```python
from build123d import *

# Parameters (mm, degrees)
SKETCH1_W           = 27
SKETCH1_H           = 10
BOSS_EXTRUDE1_DEPTH = 10
FILLET1_R           = 4
SKETCH4_R           = 8.2
CUT_EXTRUDE3_DEPTH  = 18.528548143
BOSS_EXTRUDE2_START = 2
BOSS_EXTRUDE2_DEPTH = 5.4
SKETCH2_R           = 1.7
CUT_EXTRUDE1_DEPTH  = 20.551214796
SKETCH3_R           = 3
CUT_EXTRUDE2_DEPTH  = 3


with BuildPart() as part:
    # Sketch1 → Boss-Extrude1 (new body)
    with BuildSketch(Plane.XY):
        Rectangle(SKETCH1_W, SKETCH1_H)
    extrude(amount=BOSS_EXTRUDE1_DEPTH)

    # Fillet1
    fillet1_edges = [part.edges().sort_by_distance(p)[0] for p in [
        (-13.5, 0, 10),
        (13.5, 0, 10),
        (-13.5, 0, 0),
        (13.5, 0, 0),
    ]]
    fillet(fillet1_edges, radius=FILLET1_R)

    # Sketch4 → Cut-Extrude3 (cut, through all)
    with BuildSketch(Plane(origin=(0, 0, 0), x_dir=(-1, 0, 0), z_dir=(0, 0, -1))):
        with Locations((0, -5)):
            Circle(SKETCH4_R)
    extrude(amount=-CUT_EXTRUDE3_DEPTH, mode=Mode.SUBTRACT)

    # Sketch5 → Boss-Extrude2 (add)
    with BuildSketch(Plane.XY.offset(BOSS_EXTRUDE2_START)):
        with BuildLine():
            Line((8.2, -5), (6.2, -5))
            ThreePointArc((6.2, -5), (0, 1.2), (-6.2, -5))
            Line((-6.2, -5), (-8.2, -5))
            ThreePointArc((-8.2, -5), (0, 3.2), (8.2, -5))
        make_face()
    extrude(amount=BOSS_EXTRUDE2_DEPTH)

    # Sketch2 → Cut-Extrude1 (cut, through all)
    with BuildSketch(Plane(origin=(0, 5, 0), x_dir=(1, 0, 0), z_dir=(0, 1, 0))):
        with Locations(Location((-8.5, -5, 0), (0, 0, 270))):
            Circle(SKETCH2_R)
        with Locations(Location((8.5, -5, 0), (0, 0, 270))):
            Circle(SKETCH2_R)
    extrude(amount=-CUT_EXTRUDE1_DEPTH, mode=Mode.SUBTRACT)

    # Sketch3 → Cut-Extrude2 (cut)
    with BuildSketch(Plane(origin=(0, 5, 0), x_dir=(1, 0, 0), z_dir=(0, 1, 0))):
        with Locations(Location((-8.5, -5, 0), (0, 0, 270))):
            Circle(SKETCH3_R)
        Polygon((6.887284606, -7.793305), (10.112715394, -7.793305), (11.725430787, -5), (10.112715394, -2.206695), (6.887284606, -2.206695), (5.274569213, -5), align=None)
    extrude(amount=-CUT_EXTRUDE2_DEPTH, mode=Mode.SUBTRACT)


solid = part.part
```
Geometry: final body of the model. Coordinates: model frame, mm. A direction names the side the tool comes from. Round coordinates to 2 decimals unless told otherwise and drop trailing zeros. Loops run counter-clockwise (first coordinate to the right, second up) from the corner with the lowest first, then second, coordinate; pieces in that order, holes last. Notation, with made-up numbers: (13, -36.75) -> (24, -36.75) arc R26 cw to (24, -2.75) -> close; hole circle Ø1 at (74.25, 18.5). An arc over 180 degrees is marked (long way). Write each question's results on one line, items separated by ' | '.
Item 1: Cut plane D-D on z = 5.25. Return the cut outline in (x, y), and give its area (3 significant figures).
Answers below:
outline: (-13.5, -5) -> (-10.18, -5) -> (-10.18, 2) -> (-11.49, 2) -> (-11.49, 5) -> (-13.5, 5) -> close; (-6.82, -5) -> (-6.2, -5) arc R6.2 cw to (6.2, -5) -> (6.82, -5) -> (6.82, 2) -> (5.42, 2) -> (5.42, 5) -> (-5.51, 5) -> (-5.51, 2) -> (-6.82, 2) -> close; (10.18, -5) -> (13.5, -5) -> (13.5, 5) -> (11.58, 5) -> (11.58, 2) -> (10.18, 2) -> close | area: 126 mm²
Item 2: Cut plane A-A on y = -2.25. Return the cut outline in (x, z), and give its area (3 significant figures).
Answers below:
outline: (-13.5, 4) arc R4 ccw to (-9.5, 0) -> (-7.73, 0) -> (-7.73, 2) -> (-5.56, 2) -> (-5.56, 7.4) -> (-7.73, 7.4) -> (-7.73, 10) -> (-9.5, 10) arc R4 ccw to (-13.5, 6) -> close; (5.56, 2) -> (7.73, 2) -> (7.73, 0) -> (9.5, 0) arc R4 ccw to (13.5, 4) -> (13.5, 6) arc R4 ccw to (9.5, 10) -> (7.73, 10) -> (7.73, 7.4) -> (5.56, 7.4) -> close; hole circle Ø3.4 at (-8.5, 5); hole circle Ø3.4 at (8.5, 5) | area: 107 mm²
Item 3: Pull-direction query (X, two-part tool) for faces 4 (the face through (-12.359, 0.07, 1.203)), 5 (the face through (-10, -1.5, 5.8)), 6 (the face through (7, -1.5, 5.8)), 7 (the face through (0, 5, 5)); classes: pulls with the +X half, pulls with the -X half, needs draft (parallel to the pull), parting line crosses it, or undercut.
Answers below:
face 4: pulls with the -X half | face 5: undercut | face 6: undercut | face 7: needs draft
Item 4: Cut plane B-B on x = 8.5. Return the cut outline in (y, z).
Answers below:
outline: (-5, 0) -> (5, 0) -> (5, 2.21) -> (2, 2.21) -> (2, 3.3) -> (-5, 3.3) -> close; (-5, 6.7) -> (2, 6.7) -> (2, 7.79) -> (5, 7.79) -> (5, 10) -> (-5, 10) -> close
Item 5: Set-up query: faces 1 (the face through (0.1, 1.2, 4.7)), 2 (the face through (-10.5, 2, 5)), 3 (the face through (-0.18, 3.2, 0.99)). Return all of +Z, -Z, +X, -X, +Y, -Y with unobstructed straight access to the full face (end or side cutting, diameter ignored); none if empty.
Answers below:
face 1: +Z, -Z, -Y | face 2: +Y | face 3: -Z, -Y
Item 6: Pin query (flat end, axial travel): pin 1 Ø2 at (x, z) = (8.5, 5) entering from +Y; pin 2 Ø2 at (y, z) = (1, 2) entering from -X; pin 3 Ø6 at (x, y) = (-4, -2) entering from -Z; pin 4 Ø2 at (x, y) = (-5.5, -3.5) entering from +Z. Return the tip coordinate at first contact, or that it passes through.
Answers below:
pin 1: passes through | pin 2: stops at x = -13.37 | pin 3: stops at z = 2 | pin 4: stops at z = 7.4
Item 7: Cut plane C-C on y = 3.5. Return the cut outline in (x, z), and give its area (3 significant figures).
Answers below:
outline: (-13.5, 4) arc R4 ccw to (-9.5, 0) -> (9.5, 0) arc R4 ccw to (13.5, 4) -> (13.5, 6) arc R4 ccw to (9.5, 10) -> (-9.5, 10) arc R4 ccw to (-13.5, 6) -> close; hole circle Ø6 at (-8.5, 5); hole (5.27, 5) -> (6.89, 2.21) -> (10.11, 2.21) -> (11.73, 5) -> (10.11, 7.79) -> (6.89, 7.79) -> close | area: 201 mm²
Item 8: Line query: probe 1 along X at (y, z) = (4, 3.25); probe 2 along X at (y, z) = (3.5, 7.5); probe 3 along Y at (x, z) = (10, 3). Output: solid intervals per line, ascending. Write a range as [from, to].
Answers below:
probe 1: x = [-13.43, -10.94], [-6.06, 6.28], [10.72, 13.43] | probe 2: x = [-13.21, -10.16], [-6.84, 6.72], [10.28, 13.21] | probe 3: y = [-5, 2]
